Here's how the part is built. I have some questions about the finished solid (model axes, mm). A direction names the side the tool comes from. Give positions to 0.01 mm unless a question says otherwise; leave off trailing zeros. Order: outer loops, then holes, each group sorted by start corner. A loop starts at its lowest first (then second) coordinate and runs counter-clockwise, first axis right, second up. Notation, with made-up numbers: M 40,-20.75 L 59,-20.75 A17 cw 59,-10.75 Z; hole C 77,42.25 d11. An arc over 180 degrees is marked long. Use one line per item in the form item = value.
from build123d import *

# Parameters (mm, degrees)
F0_W     = 30
F0_H     = 33.1
F1_DEPTH = 2
F2_W     = 12
F2_H     = 78


with BuildPart() as f1:
    # F0 (on Top) → F1 (new body)
    with BuildSketch(Plane.XY):
        Rectangle(F0_W, F0_H)
    extrude(amount=F1_DEPTH)

    # F2 (on Front) → F3 (revolve)
    with BuildSketch(Plane.XZ):
        with Locations((6, 41)):
            Rectangle(F2_W, F2_H)
    revolve(axis=Axis((0, 0, 40), (0, 0, 1)))

    # F4 (on Front) → F5 (revolve, cut)
    with BuildSketch(Plane.XZ):
        with BuildLine():
            Line((0, 0), (0, 80))
            Line((0, 80), (-7, 80))
            Line((-7, 80), (-7, 56.435473))
            add(Edge.make_bspline(
                [(-7, 56.435473), (-7, 43.904641), (-1, 40), (-1, 17.385136)],
                knots=[0, 0, 0, 0, 39.508592, 39.508592, 39.508592, 39.508592], degree=3))
            Line((-1, 17.385136), (-1, 0))
            Line((-1, 0), (0, 0))
        make_face()
    revolve(axis=Axis((0, 0, 40), (0, 0, -1)), mode=Mode.SUBTRACT)


solid = f1.part
Q1. I need wall thicknesses on L1, parallel to Y at x = 0, z = 12.75; L2, parallel to Y at x = 0, z = 68; L3, parallel to Z at x = 11, y = -7. Which ranges of each line are inside material? Lowest first, please.
Found:
L1 = -12 to -1, 1 to 12
L2 = -12 to -7, 7 to 12
L3 = 0 to 2
Q2. I want a section at A-A on y = 13.5. Write out the boundary of the cut face in (x, z).
Found:
outline = M -15,0 L 15,0 L 15,2 L -15,2 Z
Q3. Thinking about a two-plate mould opening in X: for faces 3 (the face through (0, 16.55, 1)), 4 (the face through (-15, 0, 1)), 5 (the face through (-6.466, -2.681, 68.053)), which applies, +X half, -X half, draft (parallel to the pull), parting line (faces both ways), or undercut?
Found:
face_3 = draft
face_4 = -X half
face_5 = undercut
Q4. I'm going to push flat-ended pins straight in: pin 1 Ø12 at (x, z) = (3, 30.5) entering from -Y; pin 2 Ø12 at (y, z) = (-7.5, 53.5) entering from +X; pin 3 Ø6 at (x, z) = (12, 22.5) entering from -Y. Where does each tip first touch, or does it pass through?
Found:
pin_1 = -12
pin_2 = 11.91
pin_3 = -7.94
Q5. On a 3-axis mill with a long thin cutter (end or side, diameter ignored), from which of +Z, -Z, +X, -X, +Y, -Y can I reach the whole of each face in a straight line? I mean faces 1 (the face through (-10, 8, 2)), 2 (the face through (-5.2, -5.2, 80)). Say none if no direction works.
Found:
face_1 = +Z
face_2 = +Z, +X, -X, +Y, -Y
